Drawing for the job (mm, zero at the part's lowest x, y, z). A direction names the side the tool comes from. Give positions to 0.01 mm unless a question says otherwise; leave off trailing zeros. Loops run counter-clockwise (first coordinate to the right, second up) from the corner with the lowest first, then second, coordinate; pieces in that order, holes last. Notation, with made-up numbers: (13.5, -24.75) -> (71.5, -24.75) arc R37 ccw to (71.5, 12.25) -> close; hole circle Ø9 at (78, 56). An arc over 180 degrees is marked (long way). Write item = value, one per line.
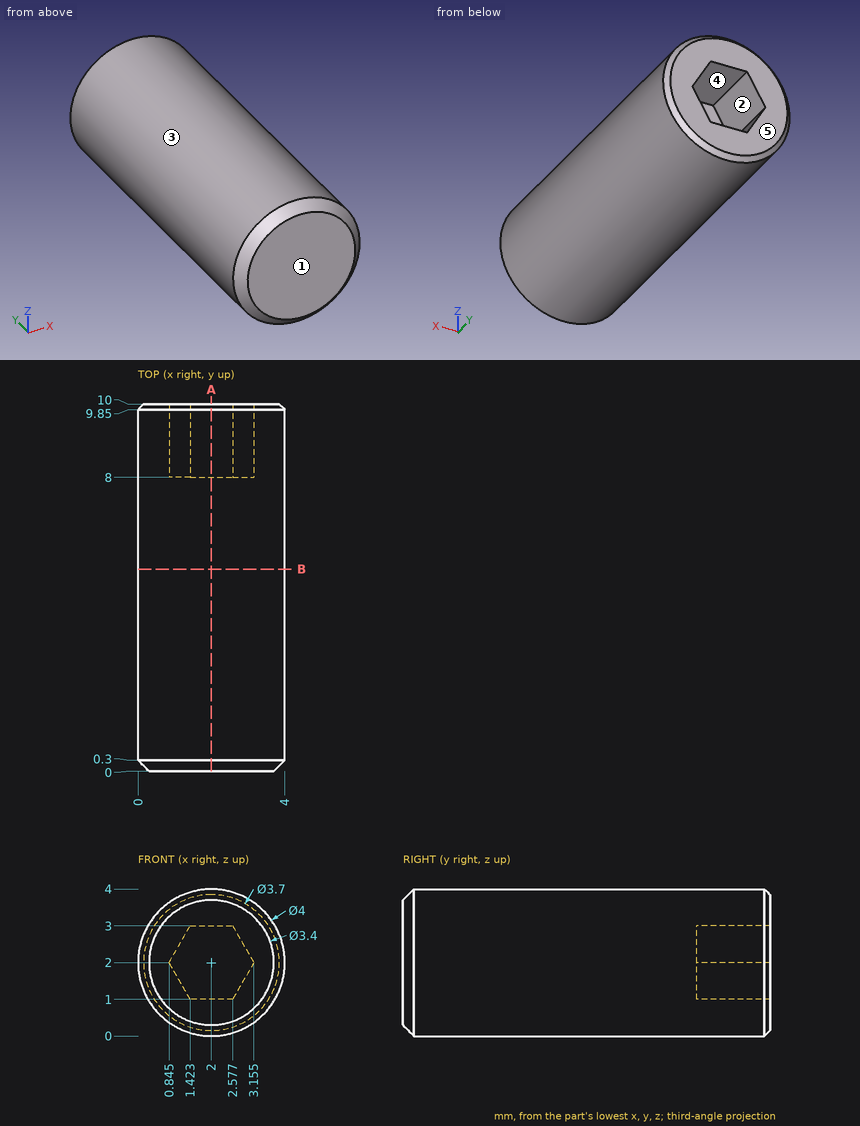
1) Which spindle directions (+Z, -Z, +X, -X, +Y, -Y) get a long thin tool onto all of the face, cutting with end or side? Do the marked faces 1 and 2. Say none if no direction does.
Resolved:
face_1 = +Z, -Z, +X, -X, -Y
face_2 = +Y
2) Drill centre lines: line 1 along Z through (x, y) = (2.05, 9); line 2 along X through (y, z) = (2.5, 2.1); line 3 along Y through (x, z) = (1.75, 2). Where is each one in solid material? Low to high. Write a range as [from, to].
Resolved:
line_1 = [0, 1], [3, 4]
line_2 = [0, 4]
line_3 = [0, 8]
3) Slice it at B-B, the plane y = 5.5. List the corners of the cut face in (x, z).
Resolved:
outline = circle Ø4 at (2, 2)
4) Pull direction X, two halves, no side cores. Call the marked faces 3, 4 and 5: pulls with the +X half, pulls with the -X half, needs draft (parallel to the pull), parting line crosses it, or undercut.
Resolved:
face_3 = parting line crosses it
face_4 = undercut
face_5 = needs draft
5) Slice it at A-A, the plane x = 2. List the corners of the cut face in (y, z).
Resolved:
outline = (0, 0.3) -> (0.3, 0) -> (9.85, 0) -> (10, 0.15) -> (10, 1) -> (8, 1) -> (8, 3) -> (10, 3) -> (10, 3.85) -> (9.85, 4) -> (0.3, 4) -> (0, 3.7) -> close
6) Drop flat-ended pins along their axis: P1, Ø1, axis at x = 2.5, z = 2, coming from the +Y side; P2, Ø1.5, axis at x = 2, z = 1.5, coming from the -Y side. Give the stop position or say it passes through.
Resolved:
P1 = 8
P2 = 0
